Could you check a few things on this model? Use its own coordinates, in mm. Face numbers are marked on the shaded views. A direction names the side the tool comes from. Give positions to 0.01 mm unless a question says otherwise; leave off trailing zeros. Loops run counter-clockwise (first coordinate to the right, second up) from the corner with the lowest first, then second, coordinate; pieces in that order, holes last.
1. Imagine slicing it at B-B (z = -19). List the corners of the cut face in (x, y) for me, plus the area to 3 significant figures.
2. Imagine slicing it at D-D (z = -63). List the corners of the cut face in (x, y) for me.
3. I need wall thicknesses on line 1 along X through (y, z) = (8.7, 34); line 2 along Z through (x, y) = (19, 3.75); line 3 along Z through (x, y) = (35, 2.25). Which ranges of each line are inside material? Lowest first, please.
4. Imagine slicing it at C-C (x = 35). List the corners of the cut face in (y, z) for me.
5. For the marked faces 1 and 2, which set-ups out of +Z, -Z, +X, -X, +Y, -Y let a thin tool reach every point of the face, with its end or its side?
6. Thinking about a two-plate mould opening in X: for the marked faces 3, 4, 5 and 6, which applies, +X half, -X half, draft (parallel to the pull), parting line (faces both ways), or undercut?
7. For P1, Ø6, axis at x = 26.5, y = 7.5, coming from the -Z side; P2, Ø6, axis at x = 35, z = -34, coming from the +Y side; P3, Ø3.5, axis at y = 8, z = -72.5, coming from the -X side, each with a flat end and sliding along its axis, tell me the tip position at first contact or that it passes through.
Autodesk Inventor part; units mm, degrees
ref_plane "YZ Plane" through (0, 0, 0) normal (1, 0, 0) x (0, 1, 0)
ref_plane "XZ Plane" through (0, 0, 0) normal (0, 1, 0) x (-1, 0, 0)
ref_plane "XY Plane" through (0, 0, 0) normal (0, 0, 1) x (1, 0, 0)
sketch "Boceto1" plane through (0, 0, 0) normal (0, 1, 0) x (-1, 0, 0)
  circle A0 centre (0, 0) radius 4.35
  line L0 (-45, 40) -> (45, 40)
  line L1 (45, 40) -> (45, -40)
  line L2 (45, -40) -> (-45, -40)
  line L3 (-45, -40) -> (-45, 40)
  line L4 (-45, 40) -> (45, -40) construction
  line L5 (45, 40) -> (-45, -40) construction
  dimension "d0" = 8.7
  dimension "d1" = 80
  dimension "d2" = 90
extrude "Extrusión1" add sketch "Boceto1" along normal blind 10
sketch "Boceto2" plane through (0, 10, 0) normal (0, 1, 0) x (1, 0, 0)
  circle A0 centre (0, 0) radius 4.35
  circle A1 centre (0, 0) radius 32.875
  dimension "d5" = 65.75
extrude "Extrusión2" cut sketch "Boceto2" against normal blind 1.4
sketch "Boceto3" plane through (0, 8.6, 0) normal (0, 1, 0) x (1, 0, 0)
  circle A0 centre (0, 0) radius 4.35
  circle A1 centre (0, 0) radius 10
  dimension "d8" = 20
extrude "Extrusión3" add sketch "Boceto3" along normal up to surface (1.4 mm away)
sketch "Boceto4" plane through (0, 8.6, 0) normal (0, 1, 0) x (1, 0, 0)
  circle A0 centre (0, -18.25) radius 2.65
  circle A1 centre (0, 18.25) radius 2.65
  point P0 (0, 0)
  dimension "d11" = 5.3
  dimension "d12" = 36.5
  dimension "d13" = 18.25
extrude "Extrusión4" [suppressed]
sketch "Boceto5" plane through (0, 8.6, 0) normal (0, 1, 0) x (1, 0, 0)
  circle A0 centre (0, -18.25) radius 2.65
  circle A1 centre (0, -18.25) radius 4.05
  circle A2 centre (0, 18.25) radius 2.65
  circle A3 centre (0, 18.25) radius 4.05
  line L0 (-4.6765, -18.25) -> (-2.3383, -14.2)
  line L1 (-2.3383, -14.2) -> (2.3383, -14.2)
  line L2 (2.3383, -14.2) -> (4.6765, -18.25)
  line L3 (4.6765, -18.25) -> (2.3383, -22.3)
  line L4 (2.3383, -22.3) -> (-2.3383, -22.3)
  line L5 (-2.3383, -22.3) -> (-4.6765, -18.25)
  line L6 (-4.6765, 18.25) -> (-2.3383, 22.3)
  line L7 (-2.3383, 22.3) -> (2.3383, 22.3)
  line L8 (2.3383, 22.3) -> (4.6765, 18.25)
  line L9 (4.6765, 18.25) -> (2.3383, 14.2)
  line L10 (2.3383, 14.2) -> (-2.3383, 14.2)
  line L11 (-2.3383, 14.2) -> (-4.6765, 18.25)
  point P0 (0, 0)
  dimension "d16" = 8.1
extrude "Extrusión5" [suppressed]
sketch "Boceto6" plane through (0, 10, 0) normal (0, 1, 0) x (1, 0, 0)
  circle A0 centre (-35, 34) radius 2.7
  circle A1 centre (35, 34) radius 2.7
  circle A2 centre (-35, -34) radius 2.7
  circle A3 centre (35, -34) radius 2.7
  line L0 (-45, 40) -> (-45, -40)
  line L1 (45, 40) -> (-45, 40)
  line L2 (-45, -40) -> (45, -40)
  line L3 (45, -40) -> (45, 40)
  point P0 (0, 0)
  dimension "d19" = 5.4
  dimension "d20" = 10
  dimension "d21" = 6
  dimension "d22" = 6
  dimension "d23" = 10
extrude "Extrusión6" cut sketch "Boceto6" against normal through all contours A0 | A1 | A2 | A3
fillet "Empalme1" radius 5 4 edges at (45, 5, 40) (45, 5, -40) (-45, 5, 40) (-45, 5, -40)
sketch "Boceto7" plane through (0, 10, 0) normal (0, 1, 0) x (1, 0, 0)
  circle A0 centre (-35, -34) radius 2.7
  circle A1 centre (-35, -34) radius 4.7
  circle A2 centre (35, -34) radius 2.7
  circle A3 centre (35, -34) radius 4.7
  circle A4 centre (35, 34) radius 2.7
  circle A5 centre (35, 34) radius 4.7
  circle A6 centre (-35, 34) radius 2.7
  circle A7 centre (-35, 34) radius 4.7
  point P0 (0, 0)
  dimension "d27" = 9.4
extrude "Extrusión7" cut sketch "Boceto7" against normal blind 2.1 contours A0 | A1 | A2 | A3 | A4 | A5 | A6 | A7
sketch "Boceto9" plane through (0, 0, 0) normal (0, -1, 0) x (1, 0, 0)
  circle A0 centre (0, 0) radius 4.35
  circle A1 centre (0, 0) radius 8.125
  dimension "d32" = 16.25
extrude "Extrusión9" cut sketch "Boceto9" against normal blind 5 contours A0 | A1
sketch "Boceto10" plane through (0, 8.6, 0) normal (0, 1, 0) x (1, 0, 0)
  circle A0 centre (19, -19) radius 2.7
  line L0 (26, 26) -> (-26, 26)
  line L1 (-26, 26) -> (-26, -26)
  line L2 (-26, -26) -> (26, -26)
  line L3 (26, -26) -> (26, 26)
  circle A1 centre (0, 0) radius 4.35
  line L4 (26, 26) -> (-26, -26) construction
  line L5 (-26, 26) -> (26, -26) construction
  circle A2 centre (0, 0) radius 10
  circle A3 centre (0, 0) radius 21
  circle A4 centre (19, -19) radius 5
  line L6 (-19, 19) -> (19, 19)
  line L7 (19, 19) -> (19, -19)
  line L8 (19, -19) -> (-19, -19)
  line L9 (-19, -19) -> (-19, 19)
  line L10 (-19, 19) -> (19, -19) construction
  line L11 (19, 19) -> (-19, -19) construction
  dimension "d35" = 52
  dimension "d36" = 52
  dimension "d37" = 42
  dimension "d38" = 5.4
  dimension "d39" = 10
  dimension "d40" = 38
extrude "Extrusión10" cut sketch "Boceto10" against normal through all contours A0 L8 L7 | L7 L8 A0
sketch "Boceto11" plane through (0, 8.6, 0) normal (0, 1, 0) x (1, 0, 0)
  circle A0 centre (19, -19) radius 2.7
  circle A1 centre (19, -19) radius 4.7
  point P0 (0, 0)
  dimension "d43" = 9.4
extrude "Extrusión11" cut sketch "Boceto11" against normal blind 2.3
pattern_circular "Patrón circular1" count 4 over 360 about axis through (0, 8.6, 0) along (0, 1, 0) of "Extrusión10", "Extrusión11"
sketch "Boceto12" plane through (0, 10, 0) normal (0, 1, 0) x (1, 0, 0)
  line L0 (40, 40) -> (-40, 40)
  line L1 (25, 40) -> (-25, 40)
  line L2 (-25, 40) -> (-25, 82)
  line L3 (-25, 82) -> (25, 82)
  line L4 (25, 82) -> (25, 40)
  point P0 (0, 0)
  point P1 (-25, 40)
  dimension "d49" = 25
  dimension "d50" = 25
  dimension "d51" = 42
extrude "Extrusión12" add sketch "Boceto12" against normal up to surface (10 mm away)
fillet "Empalme2" radius 5 4 edges at (25, 5, -40) (25, 5, -82) (-25, 5, -82) (-25, 5, -40)
sketch "Boceto13" plane through (0, 10, 0) normal (0, 1, 0) x (1, 0, 0)
  circle A0 centre (0, 53) radius 8.5
  circle A1 centre (0, 61) radius 8.5
  line L0 (-8.5, 53) -> (8.5, 53)
  line L1 (8.5, 53) -> (8.5, 61)
  line L2 (8.5, 61) -> (-8.5, 61)
  line L3 (-8.5, 61) -> (-8.5, 53)
  line L4 (20, 82) -> (-20, 82)
  point P0 (0, 0)
  point P1 (-8.5, 61)
  dimension "d55" = 17
  dimension "d56" = 21
  dimension "d57" = 8
extrude "Extrusión13" cut sketch "Boceto13" against normal through all
sketch "Boceto14" plane through (0, 10, 0) normal (0, 1, 0) x (1, 0, 0)
  circle A0 centre (-15.5, 37.5) radius 1.7
  line L0 (-17.2, 37.5) -> (-13.8, 37.5)
  line L1 (-13.8, 37.5) -> (-13.8, 45.5)
  line L2 (-13.8, 45.5) -> (-17.2, 45.5)
  line L3 (-17.2, 45.5) -> (-17.2, 37.5)
  circle A1 centre (-15.5, 45.5) radius 1.7
  arc A2 (-8.5, 53) -> (8.5, 53) centre (0, 53) ccw
  line L4 (0, 53) -> (-15.5, 53)
  line L5 (-15.5, 53) -> (-15.5, 37.5)
  line L6 (-15.5, 37.5) -> (0, 37.5)
  line L7 (0, 37.5) -> (0, 53)
  point P0 (0, 0)
  point P1 (-13.8, 45.5)
  dimension "d62" = 3.4
  dimension "d60" = 15.5
  dimension "d61" = 15.5
  dimension "d63" = 8
extrude "Extrusión14" cut sketch "Boceto14" against normal through all contours L0 A0 | L3 A1 L5 A0 | A0 L5 L0 | L0 L5 A0 | A0 L5 A1 L1 | A1 L5 L2 | L2 L5 A1 | A1 L5 L2 | L2 L5 A1
pattern_linear "Patrón rectangular1" count 2 spacing 31 along (0, 0, -1) count 2 spacing 31 along (1, 0, 0) of "Extrusión14"
sketch "Boceto15" plane through (0, 10, 0) normal (0, 1, 0) x (1, 0, 0)
  arc A0 (-17.2, 37.5) -> (-13.8, 37.5) centre (-15.5, 37.5) ccw
  line L0 (-17.2, 37.5) -> (-17.2, 45.5)
  line L1 (-13.8, 45.5) -> (-13.8, 37.5)
  arc A1 (-13.8, 45.5) -> (-17.2, 45.5) centre (-15.5, 45.5) ccw
  line L2 (-18.7, 45.5) -> (-18.7, 37.5)
  arc A2 (-18.7, 37.5) -> (-12.3, 37.5) centre (-15.5, 37.5) ccw
  line L3 (-12.3, 37.5) -> (-12.3, 45.5)
  arc A3 (-12.3, 45.5) -> (-18.7, 45.5) centre (-15.5, 45.5) ccw
  point P0 (0, 0)
  point P1 (-17.2, 28.0165)
  point P2 (-13.8, 29.8383)
  dimension "d72" = 1.5
extrude "Extrusión15" cut sketch "Boceto15" against normal blind 3 contours L0 A1 L1 A0 | A3 L3 A2 L2
pattern_linear "Patrón rectangular2" count 2 spacing 31 along (0, 0, -1) count 2 spacing 31 along (1, 0, 0) of "Extrusión15"
sketch "Boceto16" plane through (0, 10, 0) normal (0, 1, 0) x (1, 0, 0)
  circle A0 centre (-7.5, 77) radius 1.7
  circle A1 centre (7.5, 77) radius 1.7
  arc A2 (8.5, 61) -> (-8.5, 61) centre (0, 61) ccw
  line L0 (20, 82) -> (-20, 82)
  point P0 (0, 0)
  dimension "d81" = 3.4
  dimension "d82" = 15
  dimension "d83" = 7.5
  dimension "d84" = 5
extrude "Extrusión16" cut sketch "Boceto16" against normal through all
sketch "Boceto17" plane through (0, 0, 0) normal (0, -1, 0) x (1, 0, 0)
  circle A0 centre (-7.5, -77) radius 1.7
  circle A1 centre (-7.5, -77) radius 2.85
  circle A2 centre (7.5, -77) radius 1.7
  circle A3 centre (7.5, -77) radius 2.85
  line L0 (-4.2091, -77) -> (-5.8546, -79.85)
  line L1 (-5.8546, -79.85) -> (-9.1454, -79.85)
  line L2 (-9.1454, -79.85) -> (-10.7909, -77)
  line L3 (-10.7909, -77) -> (-9.1454, -74.15)
  line L4 (-9.1454, -74.15) -> (-5.8546, -74.15)
  line L5 (-5.8546, -74.15) -> (-4.2091, -77)
  line L6 (10.7909, -77) -> (9.1454, -79.85)
  line L7 (9.1454, -79.85) -> (5.8546, -79.85)
  line L8 (5.8546, -79.85) -> (4.2091, -77)
  line L9 (4.2091, -77) -> (5.8546, -74.15)
  line L10 (5.8546, -74.15) -> (9.1454, -74.15)
  line L11 (9.1454, -74.15) -> (10.7909, -77)
  point P0 (0, 0)
  dimension "d87" = 5.7
extrude "Extrusión17" cut sketch "Boceto17" against normal blind 3.1 contours A0 | A1 | A1 L5 L0 | A1 L4 L5 | L0 L1 A1 | A1 L3 L4 | L1 L2 A1 | A1 L2 L3 | A2 | A3 | A3 L11 L6 | A3 L10 L11 | L6 L7 A3 | A3 L9 L10 | L7 L8 A3 | A3 L8 L9
sketch "Boceto8" plane through (0, 10, 0) normal (0, 1, 0) x (1, 0, 0)
  line L0 (4.981, 25.0262) -> (-4.981, 25.0262)
  line L1 (-4.981, 25.0262) -> (-4.981, 54.9738)
  line L2 (-4.981, 54.9738) -> (4.981, 54.9738)
  line L3 (4.981, 54.9738) -> (4.981, 25.0262)
  line L4 (40, 40) -> (-40, 40)
  line L5 (4.981, 25.0262) -> (-4.981, 54.9738) construction
  line L6 (-4.981, 25.0262) -> (4.981, 54.9738) construction
  point P0 (0, 0)
  point P1 (0, 40)
properties part number "Shoulderbasetop"
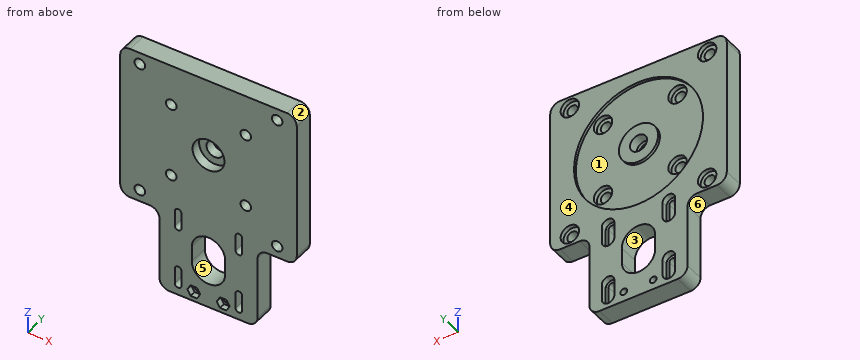
Derived:
1. outline: (-45, 0) - (-21.7, 0) - (-21.7, 6.3) - (-23.7, 6.3) - (-23.7, 8.6) - (-26.83, 8.6) - (-26.83, 10) - (-45, 10) - close; (-16.3, 0) - (16.3, 0) - (16.3, 6.3) - (14.3, 6.3) - (14.3, 8.6) - (-14.3, 8.6) - (-14.3, 6.3) - (-16.3, 6.3) - close; (21.7, 0) - (45, 0) - (45, 10) - (26.83, 10) - (26.83, 8.6) - (23.7, 8.6) - (23.7, 6.3) - (21.7, 6.3) - close
1. area: 714 mm2
2. outline: (-25, 0) - (-8.26, 0) - (-8.26, 10) - (-25, 10) - close; (8.26, 0) - (25, 0) - (25, 10) - (8.26, 10) - close
3. line 1: x = -45 to -39.7, -30.3 to 30.3, 39.7 to 45
3. line 2: z = -82 to -21.7, -16.3 to 16.3, 21.7 to 40
3. line 3: z = -40 to -36.7, -31.3 to 31.3, 36.7 to 40
4. outline: (0, -40) - (10, -40) - (10, -38.7) - (7.9, -38.7) - (7.9, -36.7) - (0, -36.7) - close; (0, -31.3) - (7.9, -31.3) - (7.9, -29.3) - (10, -29.3) - (10, 29.3) - (7.9, 29.3) - (7.9, 31.3) - (0, 31.3) - close; (0, 36.7) - (7.9, 36.7) - (7.9, 38.7) - (10, 38.7) - (10, 40) - (0, 40) - close
5. face 1: +Y
5. face 2: +Z, +X, +Y, -Y
6. face 3: undercut
6. face 4: draft
6. face 5: undercut
6. face 6: -X half
7. P1: stops at z = -80.57
7. P2: stops at y = 7.9
7. P3: stops at x = -25
